Read the model definition and answer for the solid it produces. Units are mm, in the model's axes. A direction names the side the tool comes from. Coordinates: 2 decimals unless noted, no trailing zeros. Write each loop counter-clockwise with the first axis right and the second up, starting at its lowest first coordinate (ties: lowest second). Pieces come first, ordered by that corner, then holes. Notation, with made-up numbers: (-39, 89) -> (-28, 89) arc R12 ccw to (-28, 95) -> close; hole circle Ø6 at (69, 29). An arc over 180 degrees is marked (long way). Write item = value, one per line. Start each with the question number.
1) Find the intervals of material crossed by line 1 along X through (y, z) = (0.4, 0); line 2 along X through (y, z) = (1.2, 0); line 3 along X through (y, z) = (2.8, 0), in increasing order. Write a range as from..to.
2) A tool of negligible diameter and unlimited length cuts with its end or side. For faces 1 (the face through (9.24, 1.01, -0.13)), 2 (the face through (-2.685, 2.782, -0.596)), from which of +Z, -Z, +X, -X, +Y, -Y can it reach the whole face along a straight path? Write none if from no direction.
3) Section B-B (z = 0) is taken. Determine the outline of the cut face in (x, y).
4) Section A-A (x = 0) is taken. Determine the outline of the cut face in (y, z).
5) For a pull along X with two mould halves and no side action, classify faces 3 (the face through (-3, 0, 0)), 4 (the face through (0.45, 0.25, 1.43)), 5 (the face through (3.68, 0.986, 11.684)) as released by +X, released by -X, zero draft, split by the parting line, or undercut.
6) Flat-ended cylindrical pins translate along their axes: pin 1 Ø1.5 at (x, y) = (-5, 3) entering from +Z; pin 2 Ø3 at (y, z) = (2.5, 3) entering from -X; pin 3 Ø4 at (x, z) = (8, -6.5) entering from -Y; pin 4 Ø3 at (x, z) = (0, -1) entering from +Y. Find the tip coordinate at first contact, or state that the pin passes through.
7) Section C-C (y = 1.35) is taken. Determine the outline of the cut face in (x, z).
8) Section D-D (z = -8.25) is taken. Determine the outline of the cut face in (x, y), plus the area to 3 significant figures.
from build123d import *

# Parameters (mm, degrees)
SKETCH2_R           = 12.25
BOSS_EXTRUDE1_DEPTH = 2
SKETCH3_R           = 1
CUT_EXTRUDE1_DEPTH  = 18.439180027
SKETCH4_R           = 3.75
BOSS_EXTRUDE2_DEPTH = 3
SKETCH5_R           = 1.5
CUT_EXTRUDE2_DEPTH  = 19.03122292
SKETCH6_R           = 2.75
CUT_EXTRUDE3_DEPTH  = 4.5


with BuildPart() as part:
    # Sketch2 → Boss-Extrude1 (new body)
    with BuildSketch(Plane(origin=(0, 0, 0), x_dir=(1, 0, 0), z_dir=(0, 1, 0))):
        with Locations(Location((0, 0, 0), (0, 0, 270))):
            Circle(SKETCH2_R)
    extrude(amount=BOSS_EXTRUDE1_DEPTH)

    # Sketch3 → Cut-Extrude1 (cut, through all)
    with BuildSketch(Plane(origin=(0, 2, 0), x_dir=(1, 0, 0), z_dir=(0, 1, 0))):
        with Locations(Location((0, 8.25, 0), (0, 0, 270))):
            Circle(SKETCH3_R)
        with Locations(Location((8.25, 0, 0), (0, 0, 270))):
            Circle(SKETCH3_R)
        with Locations(Location((0, -8.25, 0), (0, 0, 90))):
            Circle(SKETCH3_R)
        with Locations(Location((-8.25, 0, 0), (0, 0, 90))):
            Circle(SKETCH3_R)
    extrude(amount=-CUT_EXTRUDE1_DEPTH, mode=Mode.SUBTRACT)

    # Sketch4 → Boss-Extrude2 (add)
    with BuildSketch(Plane(origin=(0, 2, 0), x_dir=(1, 0, 0), z_dir=(0, 1, 0))):
        with Locations(Location((0, 0, 0), (0, 0, 270))):
            Circle(SKETCH4_R)
    extrude(amount=BOSS_EXTRUDE2_DEPTH)

    # Sketch5 → Cut-Extrude2 (cut, through all)
    with BuildSketch(Plane(origin=(0, 5, 0), x_dir=(1, 0, 0), z_dir=(0, 1, 0))):
        with Locations(Location((0, 0, 0), (0, 0, 270))):
            Circle(SKETCH5_R)
    extrude(amount=-CUT_EXTRUDE2_DEPTH, mode=Mode.SUBTRACT)

    # Sketch6 → Cut-Extrude3 (cut)
    with BuildSketch(Plane(origin=(0, 5, 0), x_dir=(1, 0, 0), z_dir=(0, 1, 0))):
        with Locations(Location((0, 0, 0), (0, 0, 270))):
            Circle(SKETCH6_R)
    extrude(amount=-CUT_EXTRUDE3_DEPTH, mode=Mode.SUBTRACT)


solid = part.part
Answer key:
q1.line_1 = -12.25..-9.25, -7.25..-1.5, 1.5..7.25, 9.25..12.25
q1.line_2 = -12.25..-9.25, -7.25..-2.75, 2.75..7.25, 9.25..12.25
q1.line_3 = -3.75..-2.75, 2.75..3.75
q2.face_1 = +Y, -Y
q2.face_2 = +Y
q3.outline = (-12.25, 0) -> (-9.25, 0) -> (-9.25, 2) -> (-12.25, 2) -> close; (-7.25, 0) -> (-1.5, 0) -> (-1.5, 0.5) -> (-2.75, 0.5) -> (-2.75, 5) -> (-3.75, 5) -> (-3.75, 2) -> (-7.25, 2) -> close; (1.5, 0) -> (7.25, 0) -> (7.25, 2) -> (3.75, 2) -> (3.75, 5) -> (2.75, 5) -> (2.75, 0.5) -> (1.5, 0.5) -> close; (9.25, 0) -> (12.25, 0) -> (12.25, 2) -> (9.25, 2) -> close
q4.outline = (0, -12.25) -> (2, -12.25) -> (2, -9.25) -> (0, -9.25) -> close; (0, -7.25) -> (2, -7.25) -> (2, -3.75) -> (5, -3.75) -> (5, -2.75) -> (0.5, -2.75) -> (0.5, -1.5) -> (0, -1.5) -> close; (0, 1.5) -> (0.5, 1.5) -> (0.5, 2.75) -> (5, 2.75) -> (5, 3.75) -> (2, 3.75) -> (2, 7.25) -> (0, 7.25) -> close; (0, 9.25) -> (2, 9.25) -> (2, 12.25) -> (0, 12.25) -> close
q5.face_3 = zero draft
q5.face_4 = undercut
q5.face_5 = split by the parting line
q6.pin_1 = through
q6.pin_2 = -12.15
q6.pin_3 = 0
q6.pin_4 = 0.5
q7.outline = circle Ø24.5 at (0, 0); hole circle Ø2 at (-8.25, 0); hole circle Ø5.5 at (0, 0); hole circle Ø2 at (0, -8.25); hole circle Ø2 at (0, 8.25); hole circle Ø2 at (8.25, 0)
q8.outline = (-9.06, 0) -> (-1, 0) -> (-1, 2) -> (-9.06, 2) -> close; (1, 0) -> (9.06, 0) -> (9.06, 2) -> (1, 2) -> close
q8.area = 32.2 mm^2
